Source: CAD feature listing. Evaluate the final solid. Frame: model axes, mm. Face numbers are marked on the shaded views. A direction names the side the tool comes from. Give positions to 0.01 mm unless a question says otherwise; leave off trailing zeros. Write each loop counter-clockwise with the first axis right and the second up, starting at its lowest first coordinate (ties: lowest second). Pieces come first, ordered by that corner, then holes. Notation, with made-up numbers: (-3.5, 41.25) - (26.5, 41.25) arc R19 ccw to (26.5, 62.25) - close; hole circle Ø9 at (42, 42). An arc over 180 degrees is marked (long way). One line per question, with ' | ' between items. Start each with the question number.
(1) Access query for the marked faces 4 and 5. Directions: +Z, -Z, +X, -X, +Y, -Y. A direction counts if a zero-diameter tool reaches every point of the face in a straight line with its end or side. Return the directions, or none.
(2) Section D-D, the plane z = 22. Return loops of the section in (x, y).
(3) Draft query along X for the marked faces 1, 2 and 3. Return one class per face: +X half, -X half, draft (parallel to the pull), parting line (faces both ways), or undercut.
(4) Pin query (flat end, axial travel): pin 1 (2 mm diameter, centred on x = 6, y = 5.5, fed in from -Z); pin 2 (10 mm diameter, centred on x = 10, y = 37, fed in from +Z); pin 3 (4 mm diameter, centred on x = 5.5, y = 8, fed in from +Z). Return the tip coordinate at first contact, or that it passes through.
(5) Section C-C, the plane y = 24. Return loops of the section in (x, z).
(6) Ray query, line 1 (X direction, y = 29, z = 6); line 2 (Y direction, x = -30, z = -1.1); line 3 (Z direction, x = 0, y = 4.5). Return the intervals inside material, ascending. Write a range as [from, to].
(7) Section A-A, the plane x = -6. Return loops of the section in (y, z), plus the area to 3 significant figures.
(8) Section B-B, the plane z = 1. Return loops of the section in (x, y), plus the area to 3 significant figures.
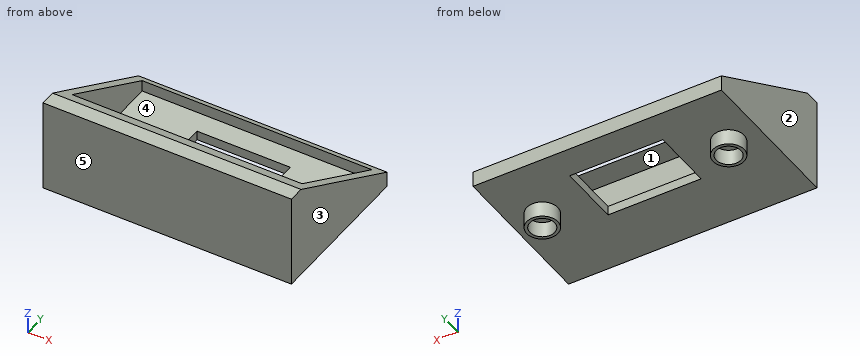
```python
from build123d import *

# Parameters (mm, degrees)
P_IDAT_VYSUNUT_M1_DEPTH  = 40
SKO_EPINA1_T             = -3
SKICA2_W                 = 30
SKICA2_H                 = 20
ODEBRAT_VYSUNUT_M1_DEPTH = 80
SKICA2_3_R               = 5
SKICA2_3_R_2             = 4
P_IDAT_VYSUNUT_M2_DEPTH  = 5


with BuildPart() as part:
    # Skica1 → P_idat vysunut_m1 (new, symmetric)
    with BuildSketch(Plane(origin=(0, 0, 0), x_dir=(0, 0, -1), z_dir=(1, 0, 0))):
        Polygon((-30, 0), (0, 0), (0, 50), (-5, 50), (-30, 5), align=None)
    extrude(amount=P_IDAT_VYSUNUT_M1_DEPTH, both=True)

    # Sko_epina1
    sko_epina1_openings = [part.faces().sort_by_distance(p)[0] for p in [
        (0, 27.5, 17.5),
    ]]
    offset(amount=SKO_EPINA1_T, openings=sko_epina1_openings, kind=Kind.INTERSECTION)

    # Skica2 → Odebrat vysunut_m1 (cut)
    with BuildSketch(Plane(origin=(0, 0, 0), x_dir=(-1, 0, 0), z_dir=(0, 0, -1))):
        with Locations((0, 30)):
            Rectangle(SKICA2_W, SKICA2_H)
    extrude(amount=-ODEBRAT_VYSUNUT_M1_DEPTH, mode=Mode.SUBTRACT)

    # Skica2<3> → P_idat vysunut_m2 (add)
    with BuildSketch(Plane(origin=(0, 0, 0), x_dir=(-1, 0, 0), z_dir=(0, 0, -1))):
        with Locations((-30, 30)):
            Circle(SKICA2_3_R)
        with Locations((-30, 30)):
            Circle(SKICA2_3_R_2, mode=Mode.SUBTRACT)
    p_idat_vysunut_m2 = extrude(amount=P_IDAT_VYSUNUT_M2_DEPTH)

    # Zrcadlit1: P_idat vysunut_m2 across plane
    add(p_idat_vysunut_m2.mirror(Plane(origin=(0, 0, 0), x_dir=(0, 0, 1), z_dir=(1, 0, 0))))


solid = part.part
```
Check sheet entries:
1) face 4: none | face 5: +Z, -Z, +X, -X, -Y
2) outline: (-40, 0) - (40, 0) - (40, 19.4) - (37, 19.4) - (37, 3) - (-37, 3) - (-37, 19.4) - (-40, 19.4) - close
3) face 1: undercut | face 2: -X half | face 3: +X half
4) pin 1: z = 0 | pin 2: z = 3 | pin 3: z = 29.44
5) outline: (-40, 0) - (-15, 0) - (-15, 3) - (-37, 3) - (-37, 19.44) - (-40, 19.44) - close; (15, 0) - (40, 0) - (40, 19.44) - (37, 19.44) - (37, 3) - (15, 3) - close
6) line 1: [-40, -37], [37, 40] | line 2: [25, 26], [34, 35] | line 3: [0, 3], [27, 30]
7) outline: (0, 0) - (20, 0) - (20, 3) - (3, 3) - (3, 27) - (10.4, 27) - (5, 30) - (0, 30) - close; (40, 0) - (50, 0) - (50, 5) - (47, 6.67) - (47, 3) - (40, 3) - close | area: 194 mm²
8) outline: (-40, 0) - (40, 0) - (40, 50) - (-40, 50) - close; hole (-15, 20) - (15, 20) - (15, 40) - (-15, 40) - close | area: 3,400 mm²
